```python
from build123d import *

# Parameters (mm, degrees)
SKETCH1_W             = 15
SKETCH1_H             = 49.5
BOSS_EXTRUDE1_DEPTH   = 3
SKETCH2_W             = 10
SKETCH2_H             = 3
SKETCH2_W_2           = 7
SKETCH2_H_2           = 10.25
SKETCH2_W_3           = 4
CUT_EXTRUDE1_DEPTH    = 27.034832437
SKETCH3_W             = 3
SKETCH3_H             = 29
BOSS_EXTRUDE2_DEPTH   = 8.25
F_3_CLEARANCE_HOLE1_D = 2.794


with BuildPart() as part:
    # Sketch1 → Boss-Extrude1 (new body)
    with BuildSketch(Plane(origin=(0, 0, 0), x_dir=(0, 0, -1), z_dir=(1, 0, 0))):
        Rectangle(SKETCH1_W, SKETCH1_H)
    extrude(amount=BOSS_EXTRUDE1_DEPTH)

    # Sketch2 → Cut-Extrude1 (cut, through all)
    with BuildSketch(Plane.ZY):
        with Locations((2.5, -23.25)):
            Rectangle(SKETCH2_W, SKETCH2_H)
        with Locations((-4, 19.625)):
            Rectangle(SKETCH2_W_2, SKETCH2_H_2)
        with Locations((5.5, 23.25)):
            Rectangle(SKETCH2_W_3, SKETCH2_H)
    extrude(amount=-CUT_EXTRUDE1_DEPTH, mode=Mode.SUBTRACT)

    # Sketch3 → Boss-Extrude2 (add)
    with BuildSketch(Plane(origin=(0, 0, -7.5), x_dir=(-1, 0, 0), z_dir=(0, 0, -1))):
        with Locations((-1.5, 0)):
            Rectangle(SKETCH3_W, SKETCH3_H)
    extrude(amount=BOSS_EXTRUDE2_DEPTH)

    # #3 Clearance Hole1 (through all)
    with Locations(Plane.ZY):
        with Locations((-7.75, 10.75), (-7.75, -10.75)):
            Hole(F_3_CLEARANCE_HOLE1_D / 2)


solid = part.part
```
Read the model definition and answer for the solid it produces. Units are mm, in the model's axes. A direction names the side the tool comes from. Coordinates: 2 decimals unless noted, no trailing zeros. Write each loop counter-clockwise with the first axis right and the second up, starting at its lowest first coordinate (ties: lowest second). Pieces come first, ordered by that corner, then holes. Notation, with made-up numbers: (-24, 58) -> (34, 58) arc R31 cw to (34, 84) -> close; hole circle Ø11 at (0.5, -20.5). An arc over 180 degrees is marked (long way). Return JSON: item names as keys, results as strings.
1. Each of these flat-tipped pins is pushed along its axis until it touches: P1, Ø1.5, axis at x = 1, z = 1, coming from the -Y side; P2, Ø0.9, axis at x = 2, y = 23.5, coming from the +Z side; P3, Ø1, axis at x = 0.5, z = -13, coming from the +Y side. Where does it stop, or does it pass through?
Found:
{"P1": "y = -21.75", "P2": "z = 3.5", "P3": "y = 14.5"}
2. A tool of negligible diameter and unlimited length cuts with its end or side. For faces 1 (the face through (1, -24.75, -5)), 2 (the face through (2, 0, -15.75)), 3 (the face through (2, -14.5, -12)), 4 (the face through (1, 23, 3.5)), 5 (the face through (1, 20, -0.5)), from which of +Z, -Z, +X, -X, +Y, -Y can it reach the whole face along a straight path? Write none if from no direction.
Found:
{"face 1": "+Z, -Z, +X, -X, -Y", "face 2": "-Z, +X, -X, +Y, -Y", "face 3": "-Z, +X, -X, -Y", "face 4": "+Z, +X, -X, +Y", "face 5": "-Z, +X, -X, +Y"}
3. A cutting plane is placed at A-A (y = 10.75). Determine the outline of the cut face in (x, z), and give its area (3 significant figures).
Found:
{"outline": "(0, -15.75) -> (3, -15.75) -> (3, -9.15) -> (0, -9.15) -> close; (0, -6.35) -> (3, -6.35) -> (3, 7.5) -> (0, 7.5) -> close", "area": "61.4 mm2"}
4. Determine the mould class of faces 6 (the face through (1, -23, -2.5)), 7 (the face through (2, 14.5, -8)), 8 (the face through (1.521, 12.135, -7.568)), 9 (the face through (1, -21.75, 2)) for opening direction Y: pulls with the +Y half, pulls with the -Y half, needs draft (parallel to the pull), parting line crosses it, or undercut.
Found:
{"face 6": "needs draft", "face 7": "pulls with the +Y half", "face 8": "undercut", "face 9": "pulls with the -Y half"}
5. Find the intervals of material crossed by line 1 along Y through (x, z) = (2.2, -7.75); line 2 along Y through (x, z) = (0.2, -2.75); line 3 along Z through (x, y) = (0.55, -20), in increasing order. Write a range as from..to.
Found:
{"line 1": "-14.5..-12.15, -9.35..9.35, 12.15..14.5", "line 2": "-24.75..14.5", "line 3": "-7.5..7.5"}
6. A cutting plane is placed at D-D (z = -11.5). Determine the outline of the cut face in (x, y).
Found:
{"outline": "(0, -14.5) -> (3, -14.5) -> (3, 14.5) -> (0, 14.5) -> close"}
7. A cutting plane is placed at B-B (x = 0.85). Determine the outline of the cut face in (y, z), and give its area (3 significant figures).
Found:
{"outline": "(-24.75, -7.5) -> (-14.5, -7.5) -> (-14.5, -15.75) -> (14.5, -15.75) -> (14.5, -0.5) -> (24.75, -0.5) -> (24.75, 3.5) -> (21.75, 3.5) -> (21.75, 7.5) -> (-21.75, 7.5) -> (-21.75, -2.5) -> (-24.75, -2.5) -> close; hole circle Ø2.79 at (-10.75, -7.75); hole circle Ø2.79 at (10.75, -7.75)", "area": "856 mm2"}
8. A cutting plane is placed at C-C (z = -8). Determine the outline of the cut face in (x, y).
Found:
{"outline": "(0, -14.5) -> (3, -14.5) -> (3, -12.12) -> (0, -12.12) -> close; (0, -9.38) -> (3, -9.38) -> (3, 9.38) -> (0, 9.38) -> close; (0, 12.12) -> (3, 12.12) -> (3, 14.5) -> (0, 14.5) -> close"}
